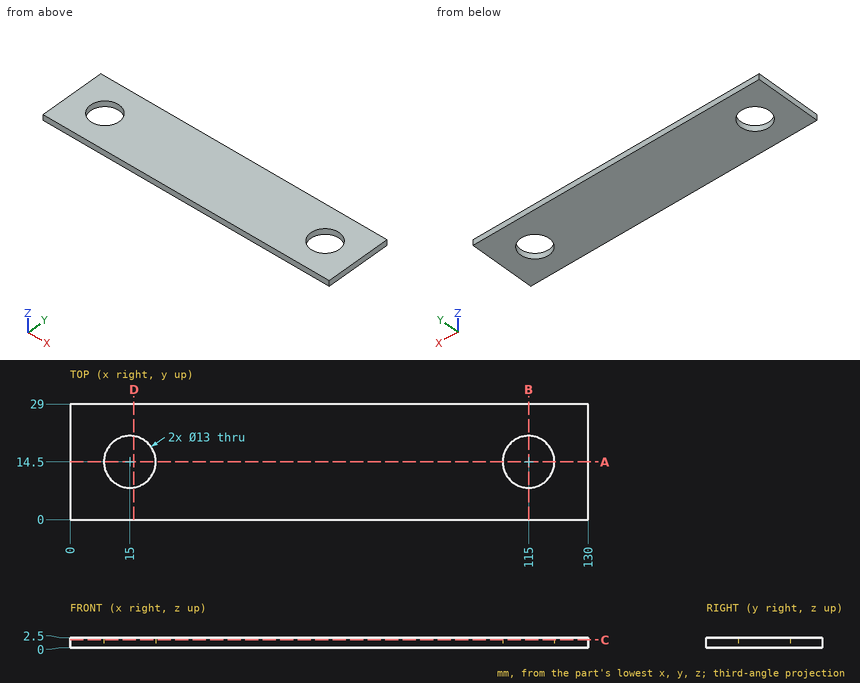
Geometry check sheet. Reference: drawing and pictorial views, mm from the part's lowest x, y, z. Give positions to 0.01 mm unless a question says otherwise; leave off trailing zeros. Order: outer loops, then holes, each group sorted by start corner. A loop starts at its lowest first (then second) coordinate and runs counter-clockwise, first axis right, second up. Notation, with made-up numbers: M 13,82 L 49,82 A13 cw 49,88 Z; hole C 51.5,57.25 d8. An arc over 180 degrees is marked long. Answer as a JSON object with one key per item and string values. Group by question number.
1) Cross-section at D-D (x = 16). Enter the section's corners in (y, z).
2) Scan lines: line 1 along Y through (x, z) = (115, 0.1); line 2 along X through (y, z) = (10.5, 2.05); line 3 along X through (y, z) = (20, 1.35). Record each from-to range of solid material in increasing order. Write a range as [from, to].
3) Cross-section at B-B (x = 115). Enter the section's corners in (y, z), then the cut area to 3 significant figures.
4) Cross-section at A-A (y = 14.5). Enter the section's corners in (x, z).
5) Cross-section at C-C (z = 1.95). Enter the section's corners in (x, y), then the cut area to 3 significant figures.
Result sheet:
{
 "1": {"outline": "M 0,0 L 8.08,0 L 8.08,2.5 L 0,2.5 Z; M 20.92,0 L 29,0 L 29,2.5 L 20.92,2.5 Z"},
 "2": {"line 1": "y = [0, 8], [21, 29]", "line 2": "x = [0, 9.88], [20.12, 109.88], [120.12, 130]", "line 3": "x = [0, 11.54], [18.46, 111.54], [118.46, 130]"},
 "3": {"outline": "M 0,0 L 8,0 L 8,2.5 L 0,2.5 Z; M 21,0 L 29,0 L 29,2.5 L 21,2.5 Z", "area": "40.0 mm2"},
 "4": {"outline": "M 0,0 L 8.5,0 L 8.5,2.5 L 0,2.5 Z; M 21.5,0 L 108.5,0 L 108.5,2.5 L 21.5,2.5 Z; M 121.5,0 L 130,0 L 130,2.5 L 121.5,2.5 Z"},
 "5": {"outline": "M 0,0 L 130,0 L 130,29 L 0,29 Z; hole C 15,14.5 d13; hole C 115,14.5 d13", "area": "3,500 mm2"}
}
